Geometry: see drawing. Coordinates: mm, zero at the bounding-box minimum. Round coordinates to 2 decimals unless told otherwise and drop trailing zeros. Loops run counter-clockwise (first coordinate to the right, second up) from the corner with the lowest first, then second, coordinate; pieces in that order, holes last. Notation, with made-up numbers: (-28.5, 20) -> (12.5, 20) arc R29 ccw to (12.5, 43) -> close; hole circle Ø7 at (-2, 37.5). An arc over 180 degrees is marked (long way). Answer in a Markdown table with one row per item.
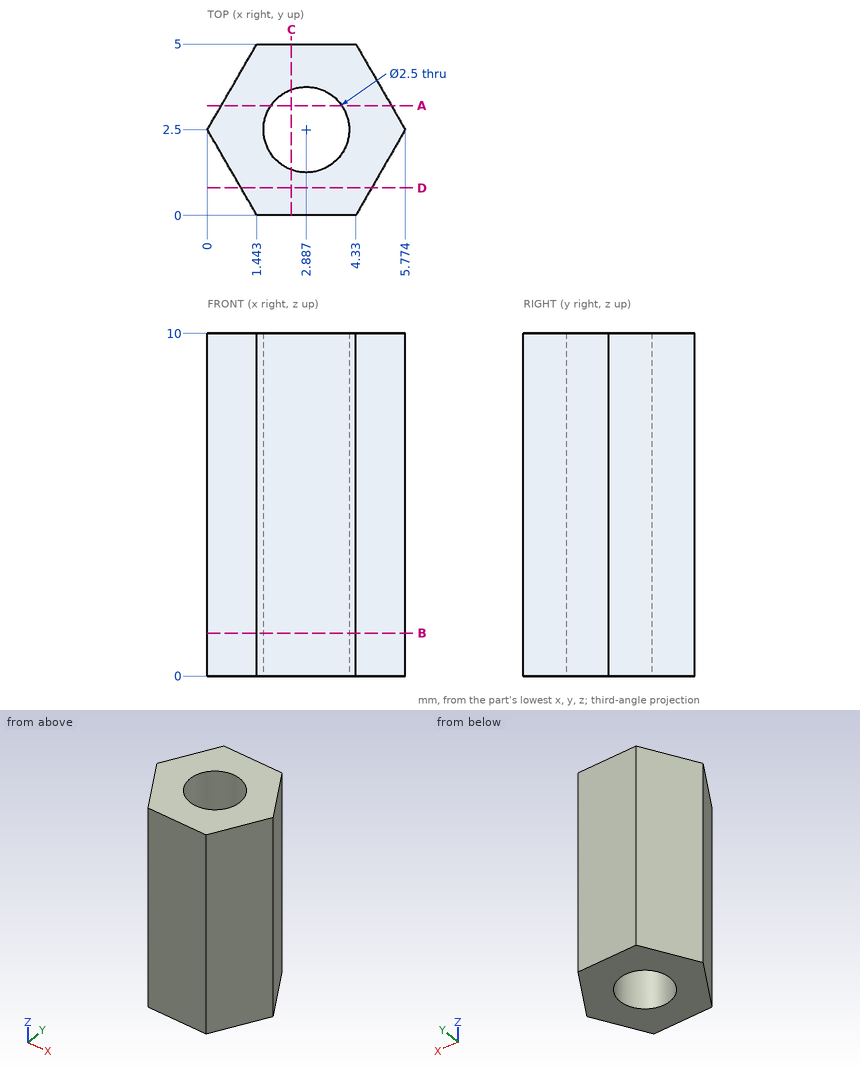
Item 1: Section query B-B, the plane z = 1.25. Output: boundary loops of the cut face in (x, y).
Ans:
| item | result |
|---|---|
| outline | (0, 2.5) -> (1.44, 0) -> (4.33, 0) -> (5.77, 2.5) -> (4.33, 5) -> (1.44, 5) -> close; hole circle Ø2.5 at (2.89, 2.5) |
Item 2: Ray query, L1, parallel to Y at x = 2.9, z = 8.25; L2, parallel to Y at x = 2.25, z = 1.25 (1 decimal); L3, parallel to X at y = 2.7, z = 8.75 (1 decimal). Return the intervals inside material, ascending.
Ans:
| item | result |
|---|---|
| L1 | 0 to 1.25, 3.75 to 5 |
| L2 | 0 to 1.4, 3.6 to 5 |
| L3 | 0.1 to 1.7, 4.1 to 5.7 |
Item 3: First-contact query: P1, Ø2, axis at y = 3, z = 4, coming from the -X side. Flat tip, straight axial feed; report the tip coordinate or a pass-through.
Ans:
| item | result |
|---|---|
| P1 | x = 0 |
Item 4: Section query D-D, the plane y = 0.8. Output: boundary loops of the cut face in (x, z), and give its area (3 significant figures).
Ans:
| item | result |
|---|---|
| outline | (0.98, 0) -> (4.79, 0) -> (4.79, 10) -> (0.98, 10) -> close |
| area | 38.1 mm2 |
Item 5: Section query C-C, the plane x = 2.45. Output: boundary loops of the cut face in (y, z).
Ans:
| item | result |
|---|---|
| outline | (0, 0) -> (1.33, 0) -> (1.33, 10) -> (0, 10) -> close; (3.67, 0) -> (5, 0) -> (5, 10) -> (3.67, 10) -> close |
Item 6: Section query A-A, the plane y = 3.2. Output: boundary loops of the cut face in (x, z).
Ans:
| item | result |
|---|---|
| outline | (0.4, 0) -> (1.85, 0) -> (1.85, 10) -> (0.4, 10) -> close; (3.92, 0) -> (5.37, 0) -> (5.37, 10) -> (3.92, 10) -> close |
